Could you check a few things on this model? Use its own coordinates, in mm. A direction names the side the tool comes from. Coordinates: 2 decimals unless noted, no trailing zeros. Write each loop counter-clockwise with the first axis right and the second up, starting at its lowest first coordinate (ties: lowest second). Pieces come first, ordered by that corner, then holes. Notation, with made-up numbers: M 28.25,50.25 L 81.25,50.25 A25 ccw 81.25,81.25 Z; hole C 52.25,86 d11. An arc over 180 degrees is marked long. Write item = value, one per line.
```python
from build123d import *

# Parameters (mm, degrees)
F_01_REMOVABLE_TWO_BOLT_NUT_KEEPER_DEPTH       = 2.4
S02_NUT_RETAINING_FACE_R                       = 7
F_02_NUT_RETAINING_FACE_DEPTH                  = 2.4
F_03_START                                     = -0.1
S03_SCREW_END_AND_TWO_M3_FASTENER_HOLE_R       = 3.6
S03_SCREW_END_AND_TWO_M3_FASTENER_HOLE_R_2     = 1.7
F_03_SCREW_END_AND_TWO_M3_FASTENER_HOLES_DEPTH = 2.6


with BuildPart() as part:
    # S01 - Removable two-bolt nut keeper → 01 - Removable two-bolt nut keeper (new body)
    with BuildSketch(Plane.XY):
        with BuildLine():
            Line((-12, 4.3), (12, 4.3))
            ThreePointArc((12, 4.3), (16.3, 0), (12, -4.3))
            Line((12, -4.3), (-12, -4.3))
            ThreePointArc((-12, -4.3), (-16.3, 0), (-12, 4.3))
        make_face()
    extrude(amount=F_01_REMOVABLE_TWO_BOLT_NUT_KEEPER_DEPTH)

    # S02 - Nut retaining face → 02 - Nut retaining face (add)
    with BuildSketch(Plane.XY):
        Circle(S02_NUT_RETAINING_FACE_R)
    extrude(amount=F_02_NUT_RETAINING_FACE_DEPTH)

    # S03 - Screw end and two M3 fastener holes → 03 - Screw end and two M3 fastener holes (cut)
    with BuildSketch(Plane.XY.offset(F_03_START)):
        with Locations(Location((0, 0, 0), (0, 0, 180))):
            Circle(S03_SCREW_END_AND_TWO_M3_FASTENER_HOLE_R)
        with Locations(Location((-12, 0, 0), (0, 0, 180))):
            Circle(S03_SCREW_END_AND_TWO_M3_FASTENER_HOLE_R_2)
        with Locations(Location((12, 0, 0), (0, 0, 180))):
            Circle(S03_SCREW_END_AND_TWO_M3_FASTENER_HOLE_R_2)
    extrude(amount=F_03_SCREW_END_AND_TWO_M3_FASTENER_HOLES_DEPTH, mode=Mode.SUBTRACT)


solid = part.part
```
Item 1: Imagine slicing it at D-D (y = -2.5). Write out the boundary of the cut face in (x, z), and give its area (3 significant figures).
Numbers:
outline = M -15.5,0 L -2.59,0 L -2.59,2.4 L -15.5,2.4 Z; M 2.59,0 L 15.5,0 L 15.5,2.4 L 2.59,2.4 Z
area = 62.0 mm²
Item 2: If I drill on line 1 along Y through (x, z) = (0, 1.5); line 2 along X through (y, z) = (1, 2.15); line 3 along Y through (x, z) = (12, 0.8), over which ranges is the centre line in solid material (lowest first)?
Numbers:
line_1 = -7 to -3.6, 3.6 to 7
line_2 = -16.18 to -13.37, -10.63 to -3.46, 3.46 to 10.63, 13.37 to 16.18
line_3 = -4.3 to -1.7, 1.7 to 4.3
Item 3: Imagine slicing it at C-C (z = 0.65). Write out the boundary of the cut face in (x, y), and give its area (3 significant figures).
Numbers:
outline = M -12,-4.3 L -5.52,-4.3 A7 ccw 5.52,-4.3 L 12,-4.3 A4.3 ccw 12,4.3 L 5.52,4.3 A7 ccw -5.52,4.3 L -12,4.3 A4.3 ccw Z; hole C -12,0 d3.4; hole C 0,0 d7.2; hole C 12,0 d3.4
area = 247 mm²
Item 4: If we mould it in two halves opening along X, with no side actions, what happens to faces 1 (the face through (-3.434, -1.081, 1.183)), 2 (the face through (-9, 4.3, 1)), 3 (the face through (-13.62, -0.51, 1.18)), 4 (the face through (16.3, 0.1, 1.2))? For each: pulls with the +X half, pulls with the -X half, needs draft (parallel to the pull), parting line crosses it, or undercut.
Numbers:
face_1 = undercut
face_2 = needs draft
face_3 = undercut
face_4 = pulls with the +X half
Item 5: For faces 5 (the face through (-9, -4.3, 1)), 6 (the face through (9, 4.3, 1)), 7 (the face through (9, -4.3, 1)), 8 (the face through (0, -7, 1)), which set-ups out of +Z, -Z, +X, -X, +Y, -Y let a thin tool reach every point of the face, with its end or its side?
Numbers:
face_5 = +Z, -Z, -X, -Y
face_6 = +Z, -Z, +X, +Y
face_7 = +Z, -Z, +X, -Y
face_8 = +Z, -Z, -Y
Item 6: Imagine slicing it at B-B (x = -1). Write out the boundary of the cut face in (y, z), and give its area (3 significant figures).
Numbers:
outline = M -6.93,0 L -3.46,0 L -3.46,2.4 L -6.93,2.4 Z; M 3.46,0 L 6.93,0 L 6.93,2.4 L 3.46,2.4 Z
area = 16.7 mm²
Item 7: I'm going to push flat-ended pins straight in: P1, Ø1.2, axis at x = 8.5, z = 1.5, coming from the +Y side; P2, Ø1.2, axis at x = 9, z = 1.5, coming from the -Y side; P3, Ø1, axis at x = 1, z = 1, coming from the +Y side. Where does each tip first touch, or does it pass through?
Numbers:
P1 = 4.3
P2 = -4.3
P3 = 6.98
Item 8: Imagine slicing it at A-A (y = 0). Write out the boundary of the cut face in (x, z).
Numbers:
outline = M -16.3,0 L -13.7,0 L -13.7,2.4 L -16.3,2.4 Z; M -10.3,0 L -3.6,0 L -3.6,2.4 L -10.3,2.4 Z; M 3.6,0 L 10.3,0 L 10.3,2.4 L 3.6,2.4 Z; M 13.7,0 L 16.3,0 L 16.3,2.4 L 13.7,2.4 Z
